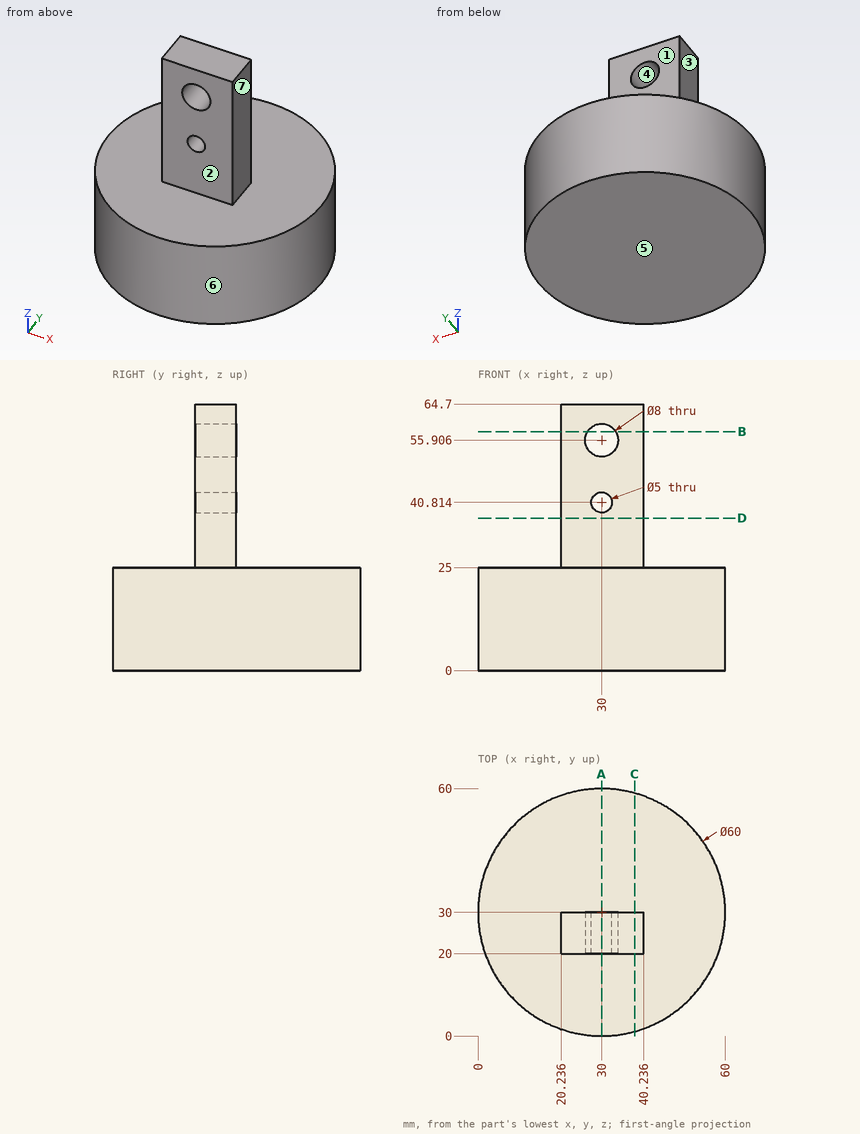
Study the drawing (mm; zero at the part's minimum x, y, z) and answer. A direction names the side the tool comes from. Give positions to 0.01 mm unless a question says otherwise; leave off trailing zeros. Loops run counter-clockwise (first coordinate to the right, second up) from the corner with the lowest first, then second, coordinate; pieces in that order, holes last. Notation, with made-up numbers: (88, 74.25) - (127, 74.25) arc R18 ccw to (127, 94.25) - close; hole circle Ø2 at (-29.75, -31.5). An arc over 180 degrees is marked (long way). Use CSV: the item, a comma, the result in double quotes. Start each with the question number.
(1) Find section B-B, the plane z = 58. Determine the outline of the cut face in (x, y), plus the area to 3 significant figures.
(2) A tool of negligible diameter and unlimited length cuts with its end or side. For the marked faces 1, 2 and 3, from which of +Z, -Z, +X, -X, +Y, -Y can it reach the whole face along a straight path? Write none if from no direction.
(3) Find the intervals of material crossed by L1, parallel to Z at x = 30, y = 23.75; L2, parallel to Z at x = 40, y = 12; L3, parallel to X at y = 21, z = 38, in increasing order.
(4) Find section D-D, the plane z = 37. Determine the outline of the cut face in (x, y).
(5) Find section A-A, the plane x = 30. Determine the outline of the cut face in (y, z).
(6) Each of these flat-tipped pins is pushed along its axis until it touches: pin 1 (12 mm diameter, centred on x = 44, z = 56.5, fed in from -Y); pin 2 (6 mm diameter, centred on x = 27.5, z = 17, fed in from +Y); pin 3 (6 mm diameter, centred on x = 26.5, z = 37.5, fed in from +Y). Where does it stop, or does it pass through?
(7) Find section C-C, the plane x = 38. Determine the outline of the cut face in (y, z), plus the area to 3 significant figures.
(8) Determine the mould class of the marked faces 4, 5, 6 and 7 for opening direction X: released by +X, released by -X, zero draft, split by the parting line, or undercut.
Results found:
1,outline,"(20.24, 20) - (26.59, 20) - (26.59, 30) - (20.24, 30) - close; (33.41, 20) - (40.24, 20) - (40.24, 30) - (33.41, 30) - close"
1,area,"132 mm^2"
2,face 1,"+Z, +X, -X, +Y"
2,face 2,"+Z, +X, -X, -Y"
2,face 3,"+Z, -X, +Y, -Y"
3,L1,"0 to 38.31, 43.31 to 51.91, 59.91 to 64.7"
3,L2,"0 to 25"
3,L3,"20.24 to 40.24"
4,outline,"(20.24, 20) - (40.24, 20) - (40.24, 30) - (20.24, 30) - close"
5,outline,"(0, 0) - (60, 0) - (60, 25) - (30, 25) - (30, 38.31) - (20, 38.31) - (20, 25) - (0, 25) - close; (20, 43.31) - (30, 43.31) - (30, 51.91) - (20, 51.91) - close; (20, 59.91) - (30, 59.91) - (30, 64.7) - (20, 64.7) - close"
6,pin 1,"y = 20"
6,pin 2,"y = 60"
6,pin 3,"y = 30"
7,outline,"(1.09, 0) - (58.91, 0) - (58.91, 25) - (30, 25) - (30, 64.7) - (20, 64.7) - (20, 25) - (1.09, 25) - close"
7,area,"1,840 mm^2"
8,face 4,"undercut"
8,face 5,"zero draft"
8,face 6,"split by the parting line"
8,face 7,"released by +X"
